Geometry check sheet. Reference: the model listing, model coordinates, mm. A direction names the side the tool comes from. Coordinates: 2 decimals unless noted, no trailing zeros. Loops run counter-clockwise (first coordinate to the right, second up) from the corner with the lowest first, then second, coordinate; pieces in that order, holes last.
from build123d import *

# Parameters (mm, degrees)
SKETCH1_W           = 14.5
SKETCH1_H           = 14.5
BOSS_EXTRUDE1_DEPTH = 7.1
SKETCH2_W           = 11.5
SKETCH2_H           = 2
CUT_EXTRUDE1_DEPTH  = 13.471367207
SKETCH5_R           = 4.7625
BOSS_EXTRUDE2_DEPTH = 1
SKETCH6_W           = 65
SKETCH6_H           = 65
BOSS_EXTRUDE3_DEPTH = 5
FILLET1_R           = 1
FILLET2_R           = 1


with BuildPart() as part:
    # Sketch1 → Boss-Extrude1 (new body)
    with BuildSketch(Plane(origin=(0, 0, 0), x_dir=(1, 0, 0), z_dir=(0, 1, 0))):
        Rectangle(SKETCH1_W, SKETCH1_H)
    extrude(amount=BOSS_EXTRUDE1_DEPTH)

    # Sketch2 → Cut-Extrude1 (cut, through all)
    with BuildSketch(Plane(origin=(0, 7.1, 0), x_dir=(1, 0, 0), z_dir=(0, 1, 0))):
        with Locations((0, -6.25)):
            Rectangle(SKETCH2_W, SKETCH2_H)
    extrude(amount=-CUT_EXTRUDE1_DEPTH, mode=Mode.SUBTRACT)

    # Sketch5 → Boss-Extrude2 (add)
    with BuildSketch(Plane.XZ):
        with Locations(Location((0, -1, 0), (0, 0, 270))):
            Circle(SKETCH5_R)
    extrude(amount=BOSS_EXTRUDE2_DEPTH)

    # Sketch6 → Boss-Extrude3 (add)
    with BuildSketch(Plane(origin=(0, 7.1, 0), x_dir=(1, 0, 0), z_dir=(0, 1, 0))):
        Rectangle(SKETCH6_W, SKETCH6_H)
    extrude(amount=BOSS_EXTRUDE3_DEPTH)

    # Fillet1
    fillet1_edges = [part.edges().sort_by_distance(p)[0] for p in [
        (32.5, 9.6, 32.5),
        (32.5, 9.6, -32.5),
        (-32.5, 9.6, -32.5),
        (-32.5, 9.6, 32.5),
    ]]
    fillet(fillet1_edges, radius=FILLET1_R)

    # Fillet2
    fillet2_edges = [part.edges().sort_by_distance(p)[0] for p in [
        (0, 7.1, 32.5),
        (0, 12.1, 32.5),
        (32.5, 7.1, 0),
        (-32.5, 7.1, 0),
        (0, 7.1, -32.5),
        (32.207106781, 7.1, 32.207106781),
        (32.207106781, 7.1, -32.207106781),
        (-32.207106781, 7.1, -32.207106781),
        (-32.207106781, 7.1, 32.207106781),
        (-32.5, 12.1, 0),
        (32.5, 12.1, 0),
        (0, 12.1, -32.5),
        (32.207106781, 12.1, 32.207106781),
        (32.207106781, 12.1, -32.207106781),
        (-32.207106781, 12.1, -32.207106781),
        (-32.207106781, 12.1, 32.207106781),
    ]]
    fillet(fillet2_edges, radius=FILLET2_R)


solid = part.part
(1) Draft check along X on faces 1 (the cylindrical face through (-2.9, -0.49, 2.78)), 2 (the flat face through (-7, 4, 7.25)), 3 (the flat face through (-5.75, 4, 6)). Enter one of: +X half, -X half, draft (parallel to the pull), parting line (faces both ways), or undercut.
Findings:
face 1: parting line
face 2: draft
face 3: undercut
(2) Sectioned sample at B-B on x = 22.5. Record the cut outline in (y, z).
Findings:
outline: (7.1, -31.5) arc R1 ccw to (8.1, -32.5) - (11.1, -32.5) arc R1 ccw to (12.1, -31.5) - (12.1, 31.5) arc R1 ccw to (11.1, 32.5) - (8.1, 32.5) arc R1 ccw to (7.1, 31.5) - close
(3) Sectioned sample at C-C on y = 6. Record the cut outline in (x, z), and give its area (3 significant figures).
Findings:
outline: (-7.25, -7.25) - (7.25, -7.25) - (7.25, 7.25) - (5.75, 7.25) - (5.75, 5.25) - (-5.75, 5.25) - (-5.75, 7.25) - (-7.25, 7.25) - close
area: 187 mm2
(4) Access from +Z, -Z, +X, -X, +Y, -Y to the whole of each face (thin tool, end or side, straight path). Record for faces 4 (the flat face through (0, 4, 5.25)), 5 (the flat face through (0, 4, -7.25)), 6 (the flat face through (7.25, 4, 0)).
Findings:
face 4: +Z, -Y
face 5: -Z, +X, -X, -Y
face 6: +Z, -Z, +X, -Y
(5) Gauge pin test, flat ends, axial feed: pin 1 Ø2 at (x, z) = (26, -11) entering from -Y; pin 2 Ø2 at (y, z) = (3.5, 6.5) entering from -X; pin 3 Ø5.5 at (x, y) = (1.5, 3.5) entering from +Z. Record the tip position at first contact, or that the pin passes through.
Findings:
pin 1: stops at y = 7.1
pin 2: stops at x = -7.25
pin 3: stops at z = 5.25
(6) Scan lines: L1, parallel to Y at x = 23, z = -24.5; L2, parallel to X at y = 4.75, z = 3; L3, parallel to X at y = 11.25, z = 26. Record each from-to range of solid material in increasing order.
Findings:
L1: y = 7.1 to 12.1
L2: x = -7.25 to 7.25
L3: x = -32.49 to 32.49
(7) Sectioned sample at A-A on z = -1. Record the cut outline in (x, y), and give its area (3 significant figures).
Findings:
outline: (-32.5, 8.1) arc R1 ccw to (-31.5, 7.1) - (-7.25, 7.1) - (-7.25, 0) - (-4.76, 0) - (-4.76, -1) - (4.76, -1) - (4.76, 0) - (7.25, 0) - (7.25, 7.1) - (31.5, 7.1) arc R1 ccw to (32.5, 8.1) - (32.5, 11.1) arc R1 ccw to (31.5, 12.1) - (-31.5, 12.1) arc R1 ccw to (-32.5, 11.1) - close
area: 437 mm2
(8) Sectioned sample at D-D on x = 0. Record the cut outline in (y, z), and give its area (3 significant figures).
Findings:
outline: (-1, -5.76) - (0, -5.76) - (0, -7.25) - (7.1, -7.25) - (7.1, -31.5) arc R1 ccw to (8.1, -32.5) - (11.1, -32.5) arc R1 ccw to (12.1, -31.5) - (12.1, 31.5) arc R1 ccw to (11.1, 32.5) - (8.1, 32.5) arc R1 ccw to (7.1, 31.5) - (7.1, 5.25) - (0, 5.25) - (0, 3.76) - (-1, 3.76) - close
area: 422 mm2
